```python
from build123d import *

# Parameters (mm, degrees)
SKETCH1_W      = 15
SKETCH1_H      = 34.5
EXTRUDE1_DEPTH = 5
SKETCH2_W      = 15
SKETCH2_H      = 5
EXTRUDE2_DEPTH = 10
SKETCH3_R      = 1.5
EXTRUDE3_DEPTH = 10
SKETCH4_R      = 1.5
EXTRUDE4_DEPTH = 10
SKETCH5_W      = 15
SKETCH5_H      = 15
EXTRUDE5_DEPTH = 0.5
EXTRUDE6_START = 0.5
SKETCH6_W      = 15
SKETCH6_H      = 10
SKETCH6_R      = 1.5
EXTRUDE6_DEPTH = 0.5


with BuildPart() as part:
    # Sketch1 → Extrude1 (new body)
    with BuildSketch(Plane(origin=(0, 0, 0), x_dir=(1, 0, 0), z_dir=(0, 1, 0))):
        Rectangle(SKETCH1_W, SKETCH1_H)
    extrude(amount=EXTRUDE1_DEPTH)

    # Sketch2 → Extrude2 (add)
    with BuildSketch(Plane(origin=(0, 5, 0), x_dir=(1, 0, 0), z_dir=(0, 1, 0))):
        with Locations((0, 14.75)):
            Rectangle(SKETCH2_W, SKETCH2_H)
    extrude(amount=EXTRUDE2_DEPTH)

    # Sketch3 → Extrude3 (cut)
    with BuildSketch(Plane(origin=(0, 5, 0), x_dir=(1, 0, 0), z_dir=(0, 1, 0))):
        with Locations(Location((0, -11.25, 0), (0, 0, 270))):
            Circle(SKETCH3_R)
    extrude(amount=-EXTRUDE3_DEPTH, mode=Mode.SUBTRACT)

    # Sketch4 → Extrude4 (cut)
    with BuildSketch(Plane.XY.offset(-12.25)):
        with Locations((0, 10)):
            Circle(SKETCH4_R)
    extrude(amount=-EXTRUDE4_DEPTH, mode=Mode.SUBTRACT)

    # Sketch5 → Extrude5 (cut)
    with BuildSketch(Plane(origin=(0, 0, -17.25), x_dir=(-1, 0, 0), z_dir=(0, 0, -1))):
        with Locations((0, 7.5)):
            Rectangle(SKETCH5_W, SKETCH5_H)
    extrude(amount=-EXTRUDE5_DEPTH, mode=Mode.SUBTRACT)

    # Sketch6 → Extrude6 (add)
    with BuildSketch(Plane.XY.offset(-12.25).offset(EXTRUDE6_START)):
        with Locations((0, 10)):
            Rectangle(SKETCH6_W, SKETCH6_H)
        with Locations((0, 10)):
            Circle(SKETCH6_R, mode=Mode.SUBTRACT)
    extrude(amount=-EXTRUDE6_DEPTH)


solid = part.part
```
Geometry check sheet. Reference: the model listing, model coordinates, mm. A direction names the side the tool comes from. Round coordinates to 2 decimals unless told otherwise and drop trailing zeros. Order: outer loops, then holes, each group sorted by start corner. A loop starts at its lowest first (then second) coordinate and runs counter-clockwise, first axis right, second up. Notation, with made-up numbers: (42.5, -12.5) - (89.5, -12.5) arc R30 ccw to (89.5, 18.5) - close; hole circle Ø10 at (-13, 0). An arc over 180 degrees is marked (long way). Use a Markdown table: item, result. Add a question column.
(1) Depth check by flat-ended pin: pin 1 (3 mm diameter, centred on x = -3, y = 11.5, fed in from +Z); pin 2 (2 mm diameter, centred on x = -5.5, z = -4, fed in from +Y). Enter the tip coordinate at first touch or a pass-through.
(2) Release check for a two-part mould opening along Y. For faces 3 (the cylindrical face through (0.07, 2.54, 9.75)), 4 (the flat face through (0, 0, 0)), 5 (the cylindrical face through (-0.325, 8.536, -14.215)), 6 (the flat face through (0, 5, 3)) record: pulls with the +Y half, pulls with the -Y half, needs draft (parallel to the pull), parting line crosses it, or undercut.
(3) Material ranges on line 1 along X through (y, z) = (1.15, 11.25); line 2 along Y through (x, z) = (0, -14.3); line 3 along Y through (x, z) = (-0.5, 3), recorded low to high. Write a range as [from, to].
(4) Sectioned sample at C-C, the plane y = 10. Enter the section's corners in (x, z).
(5) Sectioned sample at A-A, the plane x = 0. Enter the section's corners in (y, z), and give its area (3 significant figures).
(6) Tool access check on faces 1 (the flat face through (-2, 10, -11.75)), 2 (the flat face through (0, 15, -14)). Record the directions out of +Z, -Z, +X, -X, +Y, -Y that give a thin tool (end or side, any length) a straight path to the whole face; none if there is none.
(7) Sectioned sample at B-B, the plane z = 11.25. Enter the section's corners in (x, y), and give its area (3 significant figures).
(8) Sectioned sample at D-D, the plane z = -12.5. Enter the section's corners in (x, y).
Answers below:
| question | item | result |
|---|---|---|
| 1 | pin 1 | z = -11.75 |
| 1 | pin 2 | y = 5 |
| 2 | face 3 | needs draft |
| 2 | face 4 | pulls with the -Y half |
| 2 | face 5 | undercut |
| 2 | face 6 | pulls with the +Y half |
| 3 | line 1 | [-7.5, -1.5], [1.5, 7.5] |
| 3 | line 2 | [0, 8.5], [11.5, 15] |
| 3 | line 3 | [0, 5] |
| 4 | outline | (-7.5, -16.75) - (-1.5, -16.75) - (-1.5, -11.75) - (-7.5, -11.75) - close; (1.5, -16.75) - (7.5, -16.75) - (7.5, -11.75) - (1.5, -11.75) - close |
| 5 | outline | (0, -16.75) - (8.5, -16.75) - (8.5, -11.75) - (5, -11.75) - (5, 9.75) - (0, 9.75) - close; (0, 12.75) - (5, 12.75) - (5, 17.25) - (0, 17.25) - close; (11.5, -16.75) - (15, -16.75) - (15, -11.75) - (11.5, -11.75) - close |
| 5 | area | 190 mm² |
| 6 | face 1 | +Z, +X, -X, +Y |
| 6 | face 2 | +Z, -Z, +X, -X, +Y |
| 7 | outline | (-7.5, 0) - (-1.5, 0) - (-1.5, 5) - (-7.5, 5) - close; (1.5, 0) - (7.5, 0) - (7.5, 5) - (1.5, 5) - close |
| 7 | area | 60.0 mm² |
| 8 | outline | (-7.5, 0) - (7.5, 0) - (7.5, 15) - (-7.5, 15) - close; hole circle Ø3 at (0, 10) |
